from build123d import *

# Parameters (mm, degrees)
ESTRUSIONE_ESTRUSIONE2_DEPTH      = 150
ESTRUSIONE_ESTRUSIONE2_DEPTH_BACK = 150
ESTRUSIONE_ESTRUSIONE3_DEPTH      = 3.3
ESTRUSIONE_ESTRUSIONE3_DEPTH_BACK = 303.3
SCHIZZO3_W                        = 6.5
SCHIZZO3_H                        = 6.5
SCHIZZO11_W                       = 60
SCHIZZO11_H                       = 4
ESTRUSIONE_ESTRUSIONE10_DEPTH     = 2.5
ESTRUSIONE_ESTRUSIONE11_DEPTH     = 2.5
SCHIZZO11_8_W                     = 43
SCHIZZO11_8_H                     = 1.75
ESTRUSIONE_ESTRUSIONE12_DEPTH     = 4.5
SCHIZZO13_W                       = 213
SCHIZZO13_H                       = 5
ESTRUSIONE_ESTRUSIONE13_DEPTH     = 300
SCHIZZO15_W                       = 7
SCHIZZO15_H                       = 5
ESTRUSIONE_ESTRUSIONE14_DEPTH     = 4
SCHIZZO16_W                       = 213
SCHIZZO16_H                       = 5
ESTRUSIONE_ESTRUSIONE15_DEPTH     = 300
RIPETIZIONE_A_L2_COUNT            = 2
RIPETIZIONE_A_L2_PITCH            = 304
SPECCHIA2_COPY_1_SKETCH_W         = 7
SPECCHIA2_COPY_1_SKETCH_H         = 5
SPECCHIA2_COPY_1_DEPTH            = 4
SPECCHIA2_COPY_2_SKETCH_W         = 213
SPECCHIA2_COPY_2_SKETCH_H         = 5
SPECCHIA2_COPY_2_DEPTH            = 300


with BuildPart() as part:
    # Schizzo2 → Estrusione-Estrusione2 (new, two sides: drawn at the far end of the back side and taken through both)
    with BuildSketch(Plane(origin=(0, 0, 0), x_dir=(1, 0, 0), z_dir=(0, 1, 0)).offset(-ESTRUSIONE_ESTRUSIONE2_DEPTH_BACK)):
        Polygon((-113.15, 106.65), (-113.15, -106.65), (-106.65, -106.65), (-106.65, -113.15), (106.65, -113.15), (106.65, -106.65), (113.15, -106.65), (113.15, 106.65), (106.65, 106.65), (106.65, 113.15), (-106.65, 113.15), (-106.65, 106.65), align=None)
    extrude(amount=ESTRUSIONE_ESTRUSIONE2_DEPTH + ESTRUSIONE_ESTRUSIONE2_DEPTH_BACK)

    # Schizzo3 → Estrusione-Estrusione3 (add, two sides: drawn at the far end of the back side and taken through both)
    with BuildSketch(Plane.XZ.offset(150).offset(-ESTRUSIONE_ESTRUSIONE3_DEPTH_BACK)):
        with Locations((-109.9, 109.9)):
            Rectangle(SCHIZZO3_W, SCHIZZO3_H)
        with Locations((109.9, 109.9)):
            Rectangle(SCHIZZO3_W, SCHIZZO3_H)
        with Locations((109.9, -109.9)):
            Rectangle(SCHIZZO3_W, SCHIZZO3_H)
        with Locations((-109.9, -109.9)):
            Rectangle(SCHIZZO3_W, SCHIZZO3_H)
    extrude(amount=ESTRUSIONE_ESTRUSIONE3_DEPTH + ESTRUSIONE_ESTRUSIONE3_DEPTH_BACK)

    # Schizzo11 → Estrusione-Estrusione10 (add)
    with BuildSketch(Plane(origin=(0, 0, -113.15), x_dir=(-1, 0, 0), z_dir=(0, 0, -1))):
        with Locations((0, 141)):
            Rectangle(SCHIZZO11_W, SCHIZZO11_H)
    estrusione_estrusione10 = extrude(amount=ESTRUSIONE_ESTRUSIONE10_DEPTH)

    # Schizzo11_5 → Estrusione-Estrusione11 (add)
    with BuildSketch(Plane(origin=(0, 0, -113.15), x_dir=(-1, 0, 0), z_dir=(0, 0, -1))):
        Polygon((30, 139), (-30, 139), (-45, 139), (-45, 135.5), (-43, 135.5), (-43, 133.75), (0, 133.75), (43, 133.75), (43, 135.5), (45, 135.5), (45, 139), align=None)
    estrusione_estrusione11 = extrude(amount=ESTRUSIONE_ESTRUSIONE11_DEPTH)

    # Schizzo11_8 → Estrusione-Estrusione12 (add)
    with BuildSketch(Plane(origin=(0, 0, -113.15), x_dir=(-1, 0, 0), z_dir=(0, 0, -1))):
        with Locations((21.5, 132.875)):
            Rectangle(SCHIZZO11_8_W, SCHIZZO11_8_H)
        with Locations((-21.5, 132.875)):
            Rectangle(SCHIZZO11_8_W, SCHIZZO11_8_H)
        Polygon((-43, 135.5), (-45, 135.5), (-45, 132), (-43, 132), (-43, 133.75), align=None)
        Polygon((45, 132), (45, 135.5), (43, 135.5), (43, 133.75), (43, 132), align=None)
    estrusione_estrusione12 = extrude(amount=ESTRUSIONE_ESTRUSIONE12_DEPTH)

    # Schizzo13 → Estrusione-Estrusione13 (add)
    with BuildSketch(Plane(origin=(0, 0, -115.65), x_dir=(-1, 0, 0), z_dir=(0, 0, -1))):
        with Locations((-0.15, 136.25)):
            Rectangle(SCHIZZO13_W, SCHIZZO13_H)
    estrusione_estrusione13 = extrude(amount=ESTRUSIONE_ESTRUSIONE13_DEPTH)

    # Schizzo15 → Estrusione-Estrusione14 (add)
    with BuildSketch(Plane(origin=(0, 0, -415.65), x_dir=(-1, 0, 0), z_dir=(0, 0, -1))):
        with Locations((-98.15, 136.25)):
            Rectangle(SCHIZZO15_W, SCHIZZO15_H)
        with Locations((98.15, 136.25)):
            Rectangle(SCHIZZO15_W, SCHIZZO15_H)
    estrusione_estrusione14 = extrude(amount=ESTRUSIONE_ESTRUSIONE14_DEPTH)

    # Schizzo16 → Estrusione-Estrusione15 (add)
    with BuildSketch(Plane(origin=(0, 0, -419.65), x_dir=(-1, 0, 0), z_dir=(0, 0, -1))):
        with Locations((-0.15, 136.25)):
            Rectangle(SCHIZZO16_W, SCHIZZO16_H)
    estrusione_estrusione15 = extrude(amount=ESTRUSIONE_ESTRUSIONE15_DEPTH)

    # Ripetizione a L2: Estrusione-Estrusione14, Estrusione-Estrusione15 ×2
    with Locations(*[(0, 0, -i * RIPETIZIONE_A_L2_PITCH) for i in range(1, RIPETIZIONE_A_L2_COUNT)]):
        add(estrusione_estrusione14)
        add(estrusione_estrusione15)

    # Specchia2: Estrusione-Estrusione10, Estrusione-Estrusione11, Estrusione-Estrusione12, Estrusione-Estrusione13, Estrusione-Estrusione14, Estrusione-Estrusione15 across plane
    add(estrusione_estrusione10.mirror(Plane.XY))
    add(estrusione_estrusione11.mirror(Plane.XY))
    add(estrusione_estrusione12.mirror(Plane.XY))
    add(estrusione_estrusione13.mirror(Plane.XY))
    add(estrusione_estrusione14.mirror(Plane.XY))
    add(estrusione_estrusione15.mirror(Plane.XY))

    # Specchia2 copy 1 sketch → Specchia2 copy 1 (add)
    with BuildSketch(Plane(origin=(0, 0, 719.65), x_dir=(-1, 0, 0), z_dir=(0, 0, 1))):
        with Locations((-98.15, -136.25)):
            Rectangle(SPECCHIA2_COPY_1_SKETCH_W, SPECCHIA2_COPY_1_SKETCH_H)
        with Locations((98.15, -136.25)):
            Rectangle(SPECCHIA2_COPY_1_SKETCH_W, SPECCHIA2_COPY_1_SKETCH_H)
    extrude(amount=SPECCHIA2_COPY_1_DEPTH)

    # Specchia2 copy 2 sketch → Specchia2 copy 2 (add)
    with BuildSketch(Plane(origin=(0, 0, 723.65), x_dir=(-1, 0, 0), z_dir=(0, 0, 1))):
        with Locations((-0.15, -136.25)):
            Rectangle(SPECCHIA2_COPY_2_SKETCH_W, SPECCHIA2_COPY_2_SKETCH_H)
    extrude(amount=SPECCHIA2_COPY_2_DEPTH)


solid = part.part
Geometry: final body of the model. Coordinates: model frame, mm. A direction names the side the tool comes from. Give positions to 0.01 mm unless a question says otherwise; leave off trailing zeros. Write each loop counter-clockwise with the first axis right and the second up, starting at its lowest first coordinate (ties: lowest second). Pieces come first, ordered by that corner, then holes. Notation, with made-up numbers: M 43,-30 L 48,-30 A9 ccw 48,-17 Z; hole C 84.25,48 d2. An arc over 180 degrees is marked long. Answer in a Markdown table with one row per item. Add a question column.
(1) First-contact query: pin 1 (2 mm diameter, centred on x = 16.5, y = -102, fed in from -Z); pin 2 (1.5 mm diameter, centred on x = -62.5, z = 285.5, fed in from +Y); pin 3 (3.5 mm diameter, centred on x = 111.5, y = 151, fed in from +Z). Flat tips, straight axial feed; report the tip coordinate or a pass-through.
(2) Reachability of faces 1 (the flat face through (113.15, -2, 2)), 2 (the flat face through (2, 138.75, 563)), 3 (the flat face through (2, 138.75, -563)) from +Z, -Z, +X, -X, +Y, -Y: full face, straight path, thin tool, end or side. Return the list, or none.
(3) Section C-C on z = 31. Return loops of the section in (x, y), and give its area (3 significant figures).
(4) Section A-A on x = 75. Return loops of the section in (y, z).
(5) Ray query, line 1 (Z direction, x = -100, y = 135); line 2 (Y direction, x = 101.5, z = -652); line 3 (Z direction, x = -73, y = 12.5). Return the intervals inside material, ascending.
(6) Section B-B on y = 25. Return loops of the section in (x, z), and give its area (3 significant figures).
Result set:
| question | item | result |
|---|---|---|
| 1 | pin 1 | stops at z = -113.15 |
| 1 | pin 2 | stops at y = 138.75 |
| 1 | pin 3 | stops at z = 113.15 |
| 2 | face 1 | +Z, -Z, +X, +Y, -Y |
| 2 | face 2 | +Z, +X, -X, +Y |
| 2 | face 3 | -Z, +X, -X, +Y |
| 3 | outline | M -113.15,-150 L 113.15,-150 L 113.15,150 L -113.15,150 Z |
| 3 | area | 67,900 mm^2 |
| 4 | outline | M -150,-113.15 L 150,-113.15 L 150,113.15 L -150,113.15 Z; M 133.75,-1023.65 L 138.75,-1023.65 L 138.75,-723.65 L 133.75,-723.65 Z; M 133.75,-719.65 L 138.75,-719.65 L 138.75,-419.65 L 133.75,-419.65 Z; M 133.75,-415.65 L 138.75,-415.65 L 138.75,-115.65 L 133.75,-115.65 Z; M 133.75,115.65 L 138.75,115.65 L 138.75,415.65 L 133.75,415.65 Z; M 133.75,419.65 L 138.75,419.65 L 138.75,719.65 L 133.75,719.65 Z; M 133.75,723.65 L 138.75,723.65 L 138.75,1023.65 L 133.75,1023.65 Z |
| 5 | line 1 | z = -1023.65 to -115.65, -113.15 to 113.15, 115.65 to 1023.65 |
| 5 | line 2 | y = 133.75 to 138.75 |
| 5 | line 3 | z = -113.15 to 113.15 |
| 6 | outline | M -113.15,-113.15 L 113.15,-113.15 L 113.15,113.15 L -113.15,113.15 Z |
| 6 | area | 51,200 mm^2 |
